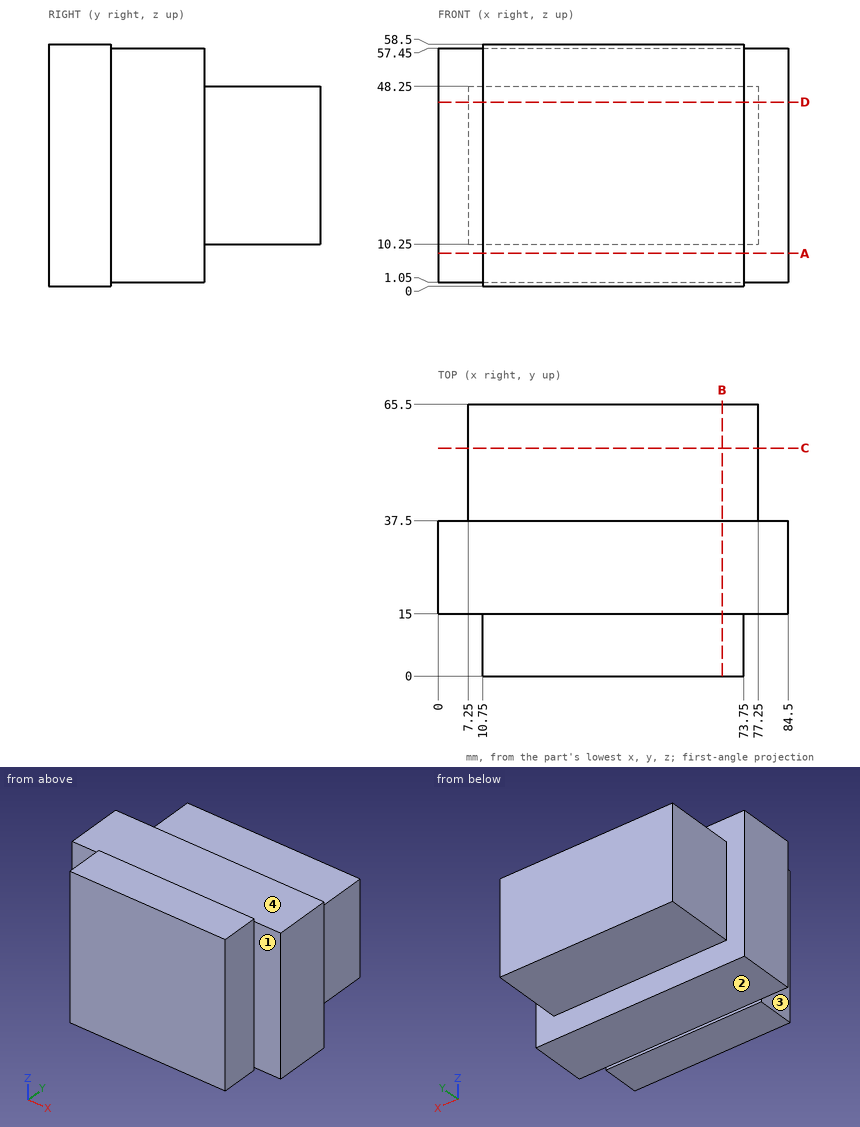
Verification items for this drawing (mm, ordinates from the low corner). A direction names the side the tool comes from. Give positions to 0.01 mm unless a question says otherwise; leave off trailing zeros. Write each loop counter-clockwise with the first axis right and the second up, starting at its lowest first coordinate (ties: lowest second). Pieces come first, ordered by that corner, then holes. Notation, with made-up numbers: (-3, 26) -> (10, 26) arc R15 ccw to (10, 52) -> close; hole circle Ø5 at (-37.75, -13). An arc over 180 degrees is marked (long way). Use one line per item in the form item = value.
Item 1: Access from +Z, -Z, +X, -X, +Y, -Y to the whole of each face (thin tool, end or side, straight path). Record for the marked faces 1, 2, 3 and 4.
Results list:
face_1 = +Z, -Z, +X, -Y
face_2 = -Z, +X, -X, +Y
face_3 = +Z, -Z, -X, -Y
face_4 = +Z, +X, -X, +Y
Item 2: Sectioned sample at C-C on y = 55. Enter the section's corners in (x, z).
Results list:
outline = (7.25, 10.25) -> (77.25, 10.25) -> (77.25, 48.25) -> (7.25, 48.25) -> close
Item 3: Sectioned sample at B-B on x = 68.5. Enter the section's corners in (y, z), plus the area to 3 significant figures.
Results list:
outline = (0, 0) -> (15, 0) -> (15, 1.05) -> (37.5, 1.05) -> (37.5, 10.25) -> (65.5, 10.25) -> (65.5, 48.25) -> (37.5, 48.25) -> (37.5, 57.45) -> (15, 57.45) -> (15, 58.5) -> (0, 58.5) -> close
area = 3,210 mm2
Item 4: Scan lines: line 1 (X direction, y = 14, z = 24.5); line 2 (Y direction, x = 9.5, z = 42); line 3 (Y direction, x = 38, z = 7). Record each from-to range of solid material in increasing order.
Results list:
line_1 = 10.75 to 73.75
line_2 = 15 to 65.5
line_3 = 0 to 37.5
Item 5: Sectioned sample at A-A on z = 8. Enter the section's corners in (x, y), plus the area to 3 significant figures.
Results list:
outline = (0, 15) -> (10.75, 15) -> (10.75, 0) -> (73.75, 0) -> (73.75, 15) -> (84.5, 15) -> (84.5, 37.5) -> (0, 37.5) -> close
area = 2,850 mm2
Item 6: Sectioned sample at D-D on z = 44.5. Enter the section's corners in (x, y), plus the area to 3 significant figures.
Results list:
outline = (0, 15) -> (10.75, 15) -> (10.75, 0) -> (73.75, 0) -> (73.75, 15) -> (84.5, 15) -> (84.5, 37.5) -> (77.25, 37.5) -> (77.25, 65.5) -> (7.25, 65.5) -> (7.25, 37.5) -> (0, 37.5) -> close
area = 4,810 mm2
Item 7: Depth check by flat-ended pin: pin 1 Ø1 at (x, y) = (74.5, 7.5) entering from +Z; pin 2 Ø25 at (x, y) = (31.5, 30) entering from +Z; pin 3 Ø7 at (x, y) = (34.5, 21) entering from -Z; pin 4 Ø14 at (x, y) = (32.5, 57) entering from +Z. Enter the tip coordinate at first touch or a pass-through.
Results list:
pin_1 = through
pin_2 = 57.45
pin_3 = 1.05
pin_4 = 48.25
